```python
from build123d import *

# Parameters (mm, degrees)
F0_W     = 76.2
F0_H     = 76.2
F1_DEPTH = 2.54
F2_W     = 76.2
F2_H     = 76.2
F2_W_2   = 71.12
F2_H_2   = 71.12
F3_DEPTH = 73.66
F5_DEPTH = 1.27


with BuildPart() as f1:
    # F0 (on Top) → F1 (new body)
    with BuildSketch(Plane.XY):
        Rectangle(F0_W, F0_H)
    extrude(amount=F1_DEPTH)

    # F2 (on face) → F3 (join)
    with BuildSketch(Plane.XY.offset(2.54)):
        Rectangle(F2_W, F2_H)
        Rectangle(F2_W_2, F2_H_2, mode=Mode.SUBTRACT)
    extrude(amount=F3_DEPTH)

    # F4 (on face) → F5 (cut)
    with BuildSketch(Plane.XZ.offset(38.1)):
        Polygon((-12.148399, 39.283356), (-25.4, 16.330909), (25.4, 16.330909), (18.117015, 28.945409), (3.810367, 36.175158), (3.810367, 48.875158), (7.764111, 46.877166), (0, 60.325), (-10.290568, 42.501213), (-5.152611, 44.375874), (-5.152611, 41.835874), align=None)
        Polygon((-33.413898, 31.524319), (-12.148399, 39.283356), (-10.290568, 42.501213), (-33.413898, 34.064319), align=None)
        Polygon((-10.290568, 42.501213), (-12.148399, 39.283356), (-5.152611, 41.835874), (-5.152611, 44.375874), align=None)
        Polygon((3.810367, 36.175158), (18.117015, 28.945409), (7.764111, 46.877166), (3.810367, 48.875158), align=None)
        Polygon((7.764111, 46.877166), (18.117015, 28.945409), (34.126167, 20.855314), (34.126167, 33.555314), align=None)
    extrude(amount=-F5_DEPTH, mode=Mode.SUBTRACT)


solid = f1.part
```
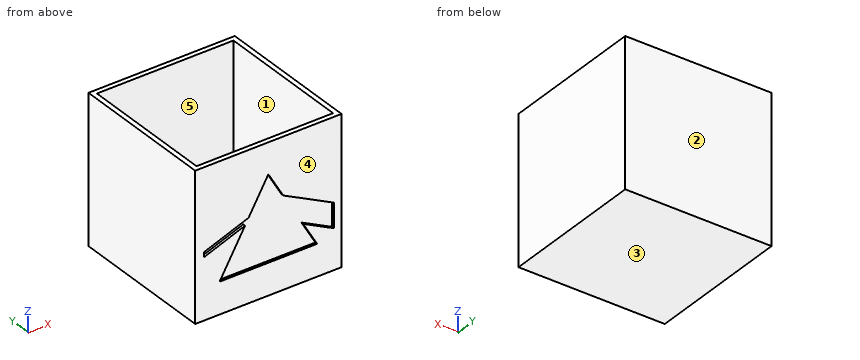
Could you check a few things on this model? Use its own coordinates, in mm. Face numbers are marked on the shaded views. A direction names the side the tool comes from. Round coordinates to 2 decimals unless told otherwise and drop trailing zeros. Loops run counter-clockwise (first coordinate to the right, second up) from the corner with the lowest first, then second, coordinate; pieces in that order, holes last. Notation, with made-up numbers: M -8.5,85.5 L 30.5,85.5 A17 ccw 30.5,89.5 Z; hole C -35.5,11 d1. An arc over 180 degrees is marked long. Put each result on its own line as item: value.
Q1. For pin 1 (1.5 mm diameter, centred on x = 4, z = 36.5, fed in from -Y); pin 2 (6 mm diameter, centred on x = 23.5, y = 28, fed in from +Z), each with a flat end and sliding along its axis, tell me the tip position at first contact or that it passes through.
Check result:
pin 1: y = -36.83
pin 2: z = 2.54
Q2. Imagine slicing it at B-B (y = 30). Write out the boundary of the cut face in (x, z), then the cut area to 3 significant figures.
Check result:
outline: M -38.1,0 L 38.1,0 L 38.1,76.2 L 35.56,76.2 L 35.56,2.54 L -35.56,2.54 L -35.56,76.2 L -38.1,76.2 Z
area: 568 mm2
Q3. I need wall thicknesses on probe 1 along Y at (x, z) = (11.5, 23); probe 2 along X at (y, z) = (-20.5, 39). Which ranges of each line are inside material? Lowest first, please.
Check result:
probe 1: -36.83 to -35.56, 35.56 to 38.1
probe 2: -38.1 to -35.56, 35.56 to 38.1
Q4. Imagine slicing it at C-C (x = 3). Write out the boundary of the cut face in (y, z).
Check result:
outline: M -38.1,0 L 38.1,0 L 38.1,76.2 L 35.56,76.2 L 35.56,2.54 L -35.56,2.54 L -35.56,76.2 L -38.1,76.2 L -38.1,55.13 L -36.83,55.13 L -36.83,16.33 L -38.1,16.33 Z
Q5. Imagine slicing it at A-A (z = 7). Write out the boundary of the cut face in (x, y).
Check result:
outline: M -38.1,-38.1 L 38.1,-38.1 L 38.1,38.1 L -38.1,38.1 Z; hole M -35.56,-35.56 L 35.56,-35.56 L 35.56,35.56 L -35.56,35.56 Z
Q6. Imagine slicing it at D-D (z = 25). Write out the boundary of the cut face in (x, y), then the cut area to 3 significant figures.
Check result:
outline: M -38.1,-38.1 L -20.39,-38.1 L -20.39,-36.83 L 20.39,-36.83 L 20.39,-38.1 L 25.92,-38.1 L 25.92,-36.83 L 34.13,-36.83 L 34.13,-38.1 L 38.1,-38.1 L 38.1,38.1 L -38.1,38.1 Z; hole M -35.56,-35.56 L 35.56,-35.56 L 35.56,35.56 L -35.56,35.56 Z
area: 686 mm2
Q7. Thinking about a two-plate mould opening in Y: for the marked faces 3, 4 and 5, which applies, released by +Y, released by -Y, zero draft, split by the parting line, or undercut?
Check result:
face 3: zero draft
face 4: released by -Y
face 5: undercut
Q8. On a 3-axis mill with a long thin cutter (end or side, diameter ignored), from which of +Z, -Z, +X, -X, +Y, -Y can I reach the whole of each face in a straight line? I mean the marked faces 1 and 2. Say none if no direction works.
Check result:
face 1: +Z
face 2: +Z, -Z, +X, -X, +Y
